```python
from build123d import *

# Parameters (mm, degrees)
F1_DEPTH = 120
F4_DEPTH = 25


with BuildPart() as f1:
    # F0 (on Top) → F1 (new body, symmetric)
    with BuildSketch(Plane.XY):
        with BuildLine():
            ThreePointArc((-62.5, 45), (-62.207107, 45.707107), (-61.5, 46))
            Line((-61.5, 46), (61.5, 46))
            ThreePointArc((61.5, 46), (62.207107, 45.707107), (62.5, 45))
            Line((62.5, 45), (62.5, -45))
            ThreePointArc((62.5, -45), (62.207107, -45.707107), (61.5, -46))
            Line((61.5, -46), (42.5, -46))
            Line((42.5, -46), (42.5, -47.5))
            Line((42.5, -47.5), (61.5, -47.5))
            ThreePointArc((61.5, -47.5), (63.267767, -46.767767), (64, -45))
            Line((64, -45), (64, 45))
            ThreePointArc((64, 45), (63.267767, 46.767767), (61.5, 47.5))
            Line((61.5, 47.5), (-61.5, 47.5))
            ThreePointArc((-61.5, 47.5), (-63.267767, 46.767767), (-64, 45))
            Line((-64, 45), (-64, -45))
            ThreePointArc((-64, -45), (-63.267767, -46.767767), (-61.5, -47.5))
            Line((-61.5, -47.5), (-42.5, -47.5))
            Line((-42.5, -47.5), (-42.5, -46))
            Line((-42.5, -46), (-61.5, -46))
            ThreePointArc((-61.5, -46), (-62.207107, -45.707107), (-62.5, -45))
            Line((-62.5, -45), (-62.5, 45))
        make_face()
    extrude(amount=F1_DEPTH, both=True)

    # F3 (on face) → F4 (cut)
    with BuildSketch(Plane(origin=(0, 47.5, 0), x_dir=(-1, 0, 0), z_dir=(0, 1, 0))):
        with BuildLine():
            Line((-25, 60), (-25, -60))
            ThreePointArc((-25, -60), (0, -85), (25, -60))
            Line((25, -60), (25, 60))
            ThreePointArc((25, 60), (0, 85), (-25, 60))
        make_face()
    extrude(amount=-F4_DEPTH, mode=Mode.SUBTRACT)


solid = f1.part
```
Geometry check sheet. Reference: the model listing, model coordinates, mm. A direction names the side the tool comes from. Give positions to 0.01 mm unless a question says otherwise; leave off trailing zeros. Loops run counter-clockwise (first coordinate to the right, second up) from the corner with the lowest first, then second, coordinate; pieces in that order, holes last. Notation, with made-up numbers: M -28,3 L 5,3 A15 ccw 5,15 Z; hole C 74,39 d7. An arc over 180 degrees is marked long. Write item = value, one per line. Start each with the question number.
1. Draft check along X on faces 4 (the face through (52, -46, 2)), 5 (the face through (52, -47.5, 2)), 6 (the face through (-52, -46, 2)), 7 (the face through (64, -1, 2)). Enter one of: +X half, -X half, draft (parallel to the pull), parting line (faces both ways), or undercut.
2. Tool access check on faces 1 (the face through (-52, -47.5, 2)), 2 (the face through (-62.5, -1, 2)), 3 (the face through (0.55, 46.76, -84.994)). Record the directions out of +Z, -Z, +X, -X, +Y, -Y that give a thin tool (end or side, any length) a straight path to the whole face; none if there is none.
3. Section check D-D, the plane z = 97. Enter the section's corners in (x, y).
4. Section check B-B, the plane y = 24.5. Enter the section's corners in (x, z).
5. Thickness scan on probe 1 along X at (y, z) = (6.5, 57); probe 2 along Y at (x, z) = (-47.5, 51); probe 3 along Y at (x, z) = (-8.5, -92). Record the ranges inside material, lowest first.
6. Go/stop test with flat-tipped pins: P1, Ø12, axis at x = 6, z = -87.5, coming from the -Y side; P2, Ø0.8, axis at y = 47, z = 1, coming from the +X side; P3, Ø0.8, axis at y = 46.5, z = -11, coming from the -X side (3 decimals). Record where each tip stops, or that it passes through.
7. Section check A-A, the plane x = 0. Enter the section's corners in (y, z).
8. Section check C-C, the plane z = 42. Enter the section's corners in (x, y), plus the area to 3 significant figures.
Values follow:
q1.face_4 = undercut
q1.face_5 = draft
q1.face_6 = undercut
q1.face_7 = +X half
q2.face_1 = +Z, -Z, +X, -X, -Y
q2.face_2 = +Z, -Z
q2.face_3 = +Y, -Y
q3.outline = M -64,-45 A2.5 ccw -61.5,-47.5 L -42.5,-47.5 L -42.5,-46 L -61.5,-46 A1 cw -62.5,-45 L -62.5,45 A1 cw -61.5,46 L 61.5,46 A1 cw 62.5,45 L 62.5,-45 A1 cw 61.5,-46 L 42.5,-46 L 42.5,-47.5 L 61.5,-47.5 A2.5 ccw 64,-45 L 64,45 A2.5 ccw 61.5,47.5 L -61.5,47.5 A2.5 ccw -64,45 Z
q4.outline = M -64,-120 L -62.5,-120 L -62.5,120 L -64,120 Z; M 62.5,-120 L 64,-120 L 64,120 L 62.5,120 Z
q5.probe_1 = -64 to -62.5, 62.5 to 64
q5.probe_2 = -47.5 to -46, 46 to 47.5
q5.probe_3 = 46 to 47.5
q6.P1 = 46
q6.P2 = 63.42
q6.P3 = -63.745
q7.outline = M 46,-120 L 47.5,-120 L 47.5,-85 L 46,-85 Z; M 46,85 L 47.5,85 L 47.5,120 L 46,120 Z
q8.outline = M -64,-45 A2.5 ccw -61.5,-47.5 L -42.5,-47.5 L -42.5,-46 L -61.5,-46 A1 cw -62.5,-45 L -62.5,45 A1 cw -61.5,46 L -25,46 L -25,47.5 L -61.5,47.5 A2.5 ccw -64,45 Z; M 25,46 L 61.5,46 A1 cw 62.5,45 L 62.5,-45 A1 cw 61.5,-46 L 42.5,-46 L 42.5,-47.5 L 61.5,-47.5 A2.5 ccw 64,-45 L 64,45 A2.5 ccw 61.5,47.5 L 25,47.5 Z
q8.area = 453 mm^2
